Model file for the job. Use its own axes, mm. Face numbers are marked on the shaded views. A direction names the side the tool comes from. Coordinates: 2 decimals unless noted, no trailing zeros. Loops run counter-clockwise (first coordinate to the right, second up) from the corner with the lowest first, then second, coordinate; pieces in that order, holes last. Notation, with made-up numbers: (11, 3) - (40, 3) arc R21 cw to (40, 26) - close; hole circle Ø9 at (-35, -38.75). An arc over 180 degrees is marked (long way). Write each question's results on one line, items separated by ' | '. Start each with the question number.
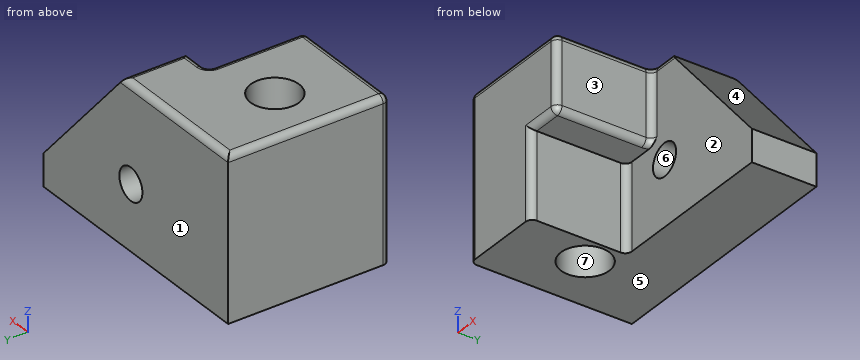
```python
from build123d import *

# Parameters (mm, degrees)
F0_W         = 203.2
F0_H         = 127
F1_DEPTH     = 127
F3_DEPTH     = 76.2
F4_SIZE2     = 101.6
F4_SIZE      = 88.9
F5_F1_R      = 5.08
F5_F2_R      = 5.08
F6_T1_DEPTH  = 66.04
F6_S5_W      = 5.1816
F6_S5_H      = 5.1816
F6_T6_DEPTH  = 5.1816
F6_T12_ANGLE = 233.2969892374
F7_R         = 12.7
F8_DEPTH     = 50.801
F9_R         = 19.05
F10_DEPTH    = 127.0010001


# Not quite as in the source:
# - a fillet or chamfer that OpenCascade refuses, or shapes differently, is made with other operations: its cross-section is extruded or revolved along the edge and cut away or added


with BuildPart() as f1:
    # F0 (on Front) → F1 (new body)
    with BuildSketch(Plane.XZ):
        with Locations((13.6157348752, 8.31202526)):
            Rectangle(F0_W, F0_H)
    extrude(amount=F1_DEPTH)

    # F2 (on face) → F3 (cut)
    with BuildSketch(Plane.XZ.offset(127)):
        Polygon((115.2157348752, 71.81202526), (5.7971677743, 71.81202526), (5.7971677743, 12.5097064301), (-22.089054808, 12.5097064301), (-22.089054808, -55.18797474), (115.2157348752, -55.18797474), align=None)
    extrude(amount=-F3_DEPTH, mode=Mode.SUBTRACT)

    # F4
    f4_edges = [f1.edges().sort_by_distance(p)[0] for p in [
        (115.215735, -25.4, 71.812025),
    ]]
    f4_side = f1.faces().sort_by_distance((-8.764887, -51.376752, 71.812025))[0]
    chamfer(f4_edges, length=F4_SIZE, length2=F4_SIZE2, reference=f4_side)

    # F5: fillet of radius 5.08 on 11 edges, made by hand

    # F5_f1
    f5_f1_edges = [f1.edges().sort_by_distance(p)[0] for p in [
        (5.7971677743, -50.8, 42.1608658451),
        (-22.089054808, -50.8, -21.3391341549),
    ]]
    fillet(f5_f1_edges, radius=F5_F1_R)

    # F5_f2
    f5_f2_edges = [f1.edges().sort_by_distance(p)[0] for p in [
        (5.7971677743, -91.44, 71.81202526),
        (5.7971677743, -127, 42.1608658451),
        (26.3157348752, -25.4, 71.81202526),
        (-30.8342651248, 0, 71.81202526),
        (-87.9842651248, -63.5, 71.81202526),
        (-8.1459435169, -127, 12.5097064301),
        (-22.089054808, -127, -21.3391341549),
        (-87.9842651248, -127, 8.31202526),
        (-41.0935486753, -127, 71.81202526),
        (7.2850653259, -52.2878975516, 71.81202526),
    ]]
    fillet(f5_f2_edges, radius=F5_F2_R)

    # F6: fillet of radius 5.08 on 2 edges, made by hand

    # F6_s2 → F6_t1 (cut)
    with BuildSketch(Plane.XZ.offset(55.88)):
        with BuildLine():
            ThreePointArc((5.7971677743, 17.5897064301), (4.3092702227, 13.9976039817), (0.7171677743, 12.5097064301))
            Line((0.7171677743, 12.5097064301), (5.7971677743, 12.5097064301))
            Line((5.7971677743, 12.5097064301), (5.7971677743, 17.5897064301))
        make_face()
    extrude(amount=F6_T1_DEPTH, mode=Mode.SUBTRACT)


with BuildPart() as f6_tool4:
    # F6_s5 → F6_t6 (new body)
    with BuildSketch(Plane.YZ.offset(0.7171677743)):
        with Locations((-124.5108, 14.9989064301)):
            Rectangle(F6_S5_W, F6_S5_H)
    extrude(amount=F6_T6_DEPTH)

    # F6_s7 → F6_t8 (revolve, cut)
    with BuildSketch(Plane(origin=(0.7171677743, -121.92, 17.5897064301), x_dir=(0, 0.7071067812, 0.7071067812), z_dir=(0, 0.7071067812, -0.7071067812))):
        with BuildLine():
            ThreePointArc((0, -5.08), (5.08, 0), (0, 5.08))
            Line((0, 5.08), (0, -5.08))
        make_face()
    revolve(axis=Axis((0.7171677743, -121.92, 17.5897064301), (1, 0, 0)), mode=Mode.SUBTRACT)


with BuildPart() as f1_1:
    add(f1.part)

    # F6_t3: cut F6_tool4
    add(f6_tool4.part, mode=Mode.SUBTRACT)


with BuildPart() as f6_tool10:
    # F6_s11 → F6_t12 (revolve)
    with BuildSketch(Plane(origin=(-19.784595187, -14.7486000708, 0), x_dir=(0, 0, 1), z_dir=(-0.8017442393, -0.5976672776, 0))):
        with BuildLine():
            ThreePointArc((17.5897064301, -56.382395344), (13.9976039817, -57.8702928955), (12.5097064301, -61.462395344))
            Line((12.5097064301, -61.462395344), (12.5097064301, -56.382395344))
            Line((12.5097064301, -56.382395344), (17.5897064301, -56.382395344))
        make_face()
    revolve(axis=Axis((10.8771677743, -55.88, 12.5097064301), (0, 0, 1)), revolution_arc=F6_T12_ANGLE)

    split(bisect_by=Plane.XZ.offset(50.8), keep=Keep.TOP)


with BuildPart() as f1_2:
    add(f1_1.part)

    # F6_t9: cut F6_tool10
    add(f6_tool10.part, mode=Mode.SUBTRACT)

    # F7 (on face) → F8 (cut, through all)
    with BuildSketch(Plane.XZ.offset(50.8)):
        with Locations((19.088730216, -4.1699022986)):
            Circle(F7_R)
    extrude(amount=-F8_DEPTH, mode=Mode.SUBTRACT)

    # F9 (on face) → F10 (cut, through all)
    with BuildSketch(Plane.XY.offset(71.81202526)):
        with Locations((-44.067915529, -68.1414976716)):
            Circle(F9_R)
    extrude(amount=-F10_DEPTH, mode=Mode.SUBTRACT)


solid = f1_2.part
```
Q1. Cut at B-B (x = -40). List the corners of the cut face in (y, z).
Q2. Which spindle directions (+Z, -Z, +X, -X, +Y, -Y) get a long thin tool onto all of the face, cutting with end or side? Do the marked faces 1, 2 and 3. Say none if no direction does.
Q3. Mould opens along X. For the marked faces 4, 5, 6 and 7 say: +X half, -X half, draft (parallel to the pull), parting line (faces both ways), or undercut.
Q4. Cut at C-C (z = 59.5). List the corners of the cut face in (x, y), and give its area (3 significant figures).
Q5. Cut at D-D (y = -29.5). List the corners of the cut face in (x, z).
Q6. Pin check, flat tips, straight feed: pin 1 (3 mm diameter, centred on y = -69, z = 32, fed in from +X); pin 2 (12 mm diameter, centred on x = -15.5, y = -80.5, fed in from -Z). Stop position of each tip, or through.
Q7. Drill centre lines: L1, parallel to Z at x = 20, y = -37; L2, parallel to X at y = -108.5, z = 5; L3, parallel to Z at x = -15, y = -118.5. Where is each one in solid material? Low to high. Write a range as from..to.
Q8. Cut at A-A (y = -72.5). List the corners of the cut face in (x, z).
Check result:
1) outline: (-127, -55.19) - (-86.75, -55.19) - (-86.75, 71.81) - (-121.92, 71.81) arc R5.08 ccw to (-127, 66.73) - close; (-49.53, -55.19) - (0, -55.19) - (0, 66.73) arc R5.08 ccw to (-5.08, 71.81) - (-49.53, 71.81) - close
2) face 1: +Z, -Z, +X, -X, +Y | face 2: -Z, +X, -Y | face 3: +Z, -Z, +X, -Y
3) face 4: +X half | face 5: draft | face 6: undercut | face 7: undercut
4) outline: (-87.98, -121.92) arc R5.08 ccw to (-82.9, -127) - (0.72, -127) arc R5.08 ccw to (5.8, -121.92) - (5.8, -55.88) arc R5.08 cw to (10.88, -50.8) - (37.09, -50.8) - (37.09, 0) - (-87.98, 0) - close; hole circle Ø38.1 at (-44.07, -68.14) | area: 12,400 mm²
5) outline: (-87.98, -55.19) - (115.22, -55.19) - (115.22, -29.79) - (27.83, 70.08) arc R5.08 ccw to (24.01, 71.81) - (-82.9, 71.81) arc R5.08 ccw to (-87.98, 66.73) - close; hole circle Ø25.4 at (19.09, -4.17)
6) pin 1: x = 5.8 | pin 2: z = 12.51
7) L1: -55.19..-16.84, 8.5..71.81 | L2: -87.98..-22.09 | L3: 12.51..71.81
8) outline: (-87.98, -55.19) - (-62.61, -55.19) - (-62.61, 71.81) - (-82.9, 71.81) arc R5.08 ccw to (-87.98, 66.73) - close; (-25.52, -55.19) - (-22.09, -55.19) - (-22.09, 12.51) - (0.72, 12.51) arc R5.08 ccw to (5.8, 17.59) - (5.8, 66.73) arc R5.08 ccw to (0.72, 71.81) - (-25.52, 71.81) - close
